Source: CAD feature listing. Evaluate the final solid. Frame: model axes, mm. A direction names the side the tool comes from. Give positions to 0.01 mm unless a question says otherwise; leave off trailing zeros. Order: outer loops, then holes, each group sorted by start corner. A loop starts at its lowest first (then second) coordinate and runs counter-clockwise, first axis right, second up. Notation, with made-up numbers: M 52,70.25 L 88,70.25 A11 ccw 88,83.25 Z; hole C 81.25,-11 d6. An arc over 180 degrees is marked long. Use CSV: the item, a comma, the result in double quotes. Start each with the question number.
1. Mould query, pull axis X, two halves, no side actions, for faces 4 (the flat face through (-57.728, -87.952, 6.439)), 5 (the flat face through (0, -170, 6)), 6 (the cylindrical face through (38.752, 0.099, 6.383)). Classes: released by +X, released by -X, zero draft, split by the parting line, or undercut.
2. Section query D-D, the plane y = 49. Return the cut outline in (x, z), plus the area to 3 significant figures.
3. Section query C-C, the plane x = 70. Return the cut outline in (y, z).
4. Line query: line 1 along Z through (x, y) = (10, -39.5); line 2 along Y through (x, z) = (-32.5, 7.5); line 3 along X through (y, z) = (-33.5, 12). Output: solid intervals per line, ascending. Write a range as [from, to].
5. Pin query (flat end, axial travel): P1, Ø2.5, axis at x = -30, y = -28, coming from the -Z side; P2, Ø9, axis at x = -41, y = 0, coming from the +Z side; P3, Ø4, axis at y = -140.5, z = 4.5, coming from the +X side; P4, Ø4, axis at y = -27, z = 8.5, coming from the -X side. Return the tip coordinate at first contact, or that it passes through.
6. Section query B-B, the plane x = 50. Return the cut outline in (y, z).
7. Reachability of faces 1 (the flat face through (39, -2, 4)), 2 (the cylindrical face through (31.14, -28.32, 6.38)), 3 (the flat face through (19, -19, 8.7)) from +Z, -Z, +X, -X, +Y, -Y: full face, straight path, thin tool, end or side. Return the list, or none.
8. Section query A-A, the plane y = -108. Return the cut outline in (x, z).
from build123d import *

# Parameters (mm, degrees)
BOSS_EXTRUDE1_DEPTH            = 12.7
CUT_EXTRUDE1_DEPTH             = 187.242556898
M8_CLEARANCE_HOLE1_D           = 9
M8_CLEARANCE_HOLE1_DEPTH       = 25.4
M8_CLEARANCE_HOLE1_TIP         = 2.703872786
M4X0_7_TAPPED_HOLE1_D          = 3.3
M4_CLEARANCE_HOLE1_D           = 4.8
HOLE2_D                        = 51
HOLE2_CBORE_D                  = 88.9
HOLE2_CBORE_DEPTH              = 4
CBORE_FOR_M4_SHCS1_D           = 4.5
CBORE_FOR_M4_SHCS1_CBORE_D     = 8
CBORE_FOR_M4_SHCS1_CBORE_DEPTH = 4
FILLET1_R                      = 10


with BuildPart() as part:
    # Sketch1 → Boss-Extrude1 (new body)
    with BuildSketch(Plane.XY.offset(12.7)):
        with BuildLine():
            Line((40, -170), (73.308387301, -15.839202988))
            ThreePointArc((73.308387301, -15.839202988), (0, 75), (-73.308387301, -15.839202988))
            Line((-73.308387301, -15.839202988), (-40, -170))
            Line((-40, -170), (40, -170))
        make_face()
    extrude(amount=-BOSS_EXTRUDE1_DEPTH)

    # Sketch2 → Cut-Extrude1 (cut, through all)
    with BuildSketch(Plane(origin=(0, 0, 0), x_dir=(-1, 0, 0), z_dir=(0, 0, -1))):
        with BuildLine():
            Line((-18.5, -124), (-18.5, -134))
            ThreePointArc((-18.5, -134), (0, -152.5), (18.5, -134))
            Line((18.5, -134), (18.5, -124))
            ThreePointArc((18.5, -124), (0, -105.5), (-18.5, -124))
        make_face()
    extrude(amount=-CUT_EXTRUDE1_DEPTH, mode=Mode.SUBTRACT)

    # M8 Clearance Hole1
    with Locations(Plane(origin=(0, 0, 0), x_dir=(-1, 0, 0), z_dir=(0, 0, -1))):
        with Locations((-50, -60), (50, -60), (-50, 40), (50, 40)):
            Hole(M8_CLEARANCE_HOLE1_D / 2, depth=M8_CLEARANCE_HOLE1_DEPTH)
            with Locations((0, 0, -(M8_CLEARANCE_HOLE1_DEPTH + M8_CLEARANCE_HOLE1_TIP / 2))):  # 118° drill point
                Cone(0, M8_CLEARANCE_HOLE1_D / 2, M8_CLEARANCE_HOLE1_TIP, mode=Mode.SUBTRACT)

    # M4x0.7 Tapped Hole1 (through all)
    with Locations(Plane.XY.offset(12.7)):
        with Locations((-25.5, -116.75), (-25.5, -141.25), (25.5, -116.75), (25.5, -141.25)):
            Hole(M4X0_7_TAPPED_HOLE1_D / 2)

    # M4 Clearance Hole1 (through all)
    with Locations(Plane.XY.offset(12.7)):
        with Locations((70, 0), (-70, 0)):
            Hole(M4_CLEARANCE_HOLE1_D / 2)

    # Hole2 (through all)
    with Locations(Plane.XY.offset(12.7)):
        with Locations((0, 0)):
            CounterBoreHole(HOLE2_D / 2, HOLE2_CBORE_D / 2, HOLE2_CBORE_DEPTH)

    # CBORE for M4 SHCS1 (through all)
    with Locations(Plane(origin=(0, 0, 0), x_dir=(-1, 0, 0), z_dir=(0, 0, -1))):
        with Locations((28.991378029, 28.991378029), (41, 0), (28.991378029, -28.991378029), (0, -41), (-28.991378029, -28.991378029), (-41, 0), (-28.991378029, 28.991378029), (0, 41)):
            CounterBoreHole(CBORE_FOR_M4_SHCS1_D / 2, CBORE_FOR_M4_SHCS1_CBORE_D / 2, CBORE_FOR_M4_SHCS1_CBORE_DEPTH)

    # Fillet1
    fillet1_edges = [part.edges().sort_by_distance(p)[0] for p in [
        (-40, -170, 6.35),
        (40, -170, 6.35),
    ]]
    fillet(fillet1_edges, radius=FILLET1_R)


solid = part.part
Result set:
1,face 4,"released by -X"
1,face 5,"zero draft"
1,face 6,"undercut"
2,outline,"M -56.78,0 L 56.78,0 L 56.78,12.7 L -56.78,12.7 Z"
2,area,"1,440 mm2"
3,outline,"M -31.15,0 L -2.4,0 L -2.4,12.7 L -31.15,12.7 Z; M 2.4,0 L 26.93,0 L 26.93,12.7 L 2.4,12.7 Z"
4,line 1,"[0, 8.7]"
4,line 2,"[-169.98, 67.59]"
4,line 3,"[-69.49, -29.22], [29.22, 69.49]"
5,P1,"z = 4"
5,P2,"z = 12.7"
5,P3,"x = 46.81"
5,P4,"x = -71.33"
6,outline,"M -123.72,0 L -64.5,0 L -64.5,12.7 L -123.72,12.7 Z; M -55.5,0 L 35.5,0 L 35.5,12.7 L -55.5,12.7 Z; M 44.5,0 L 55.9,0 L 55.9,12.7 L 44.5,12.7 Z"
7,face 1,"-Z"
7,face 2,"+Z, -Z"
7,face 3,"+Z"
8,outline,"M -53.4,0 L -9.29,0 L -9.29,12.7 L -53.4,12.7 Z; M 9.29,0 L 53.4,0 L 53.4,12.7 L 9.29,12.7 Z"
